Design review of the part shown in the three views and the two pictorial views. Dimensions are in mm from the part's minimum x, y and z. A direction names the side the tool comes from. Coordinates: 2 decimals unless noted, no trailing zeros. Loops run counter-clockwise (first coordinate to the right, second up) from the corner with the lowest first, then second, coordinate; pieces in that order, holes last. Notation, with made-up numbers: M 3,-6.75 L 22,-6.75 A12 ccw 22,16.25 Z; hole C 68.25,65.25 d4. An arc over 180 degrees is marked long. Answer as a JSON object with one key per item and string values. Group by question number.
Item 1: Mouldability with a two-part tool opening along X and no side actions: class the marked faces 3, 4, 5 and 6 as +X half, -X half, draft (parallel to the pull), parting line (faces both ways), or undercut.
Item 2: Add section A-A (x = 237). State the section outline as (y, z) points, then the cut area to 3 significant figures.
Item 3: Tool access review of the marked faces 1 and 2: name each direction out of +Z, -Z, +X, -X, +Y, -Y from which nothing blocks a thin tool from reaching the whole face with its end or side.
Item 4: Wall thickness on L1, parallel to X at y = 83, z = 149.5; L2, parallel to Y at x = 105, z = 110: over which ranges is each line inside the solid? List them lowest first. Write a range as from..to.
Item 5: Add section B-B (y = 100). State the section outline as (x, z) points, then the cut area to 3 significant figures.
Item 6: Add section C-C (z = 172). State the section outline as (x, y) points.
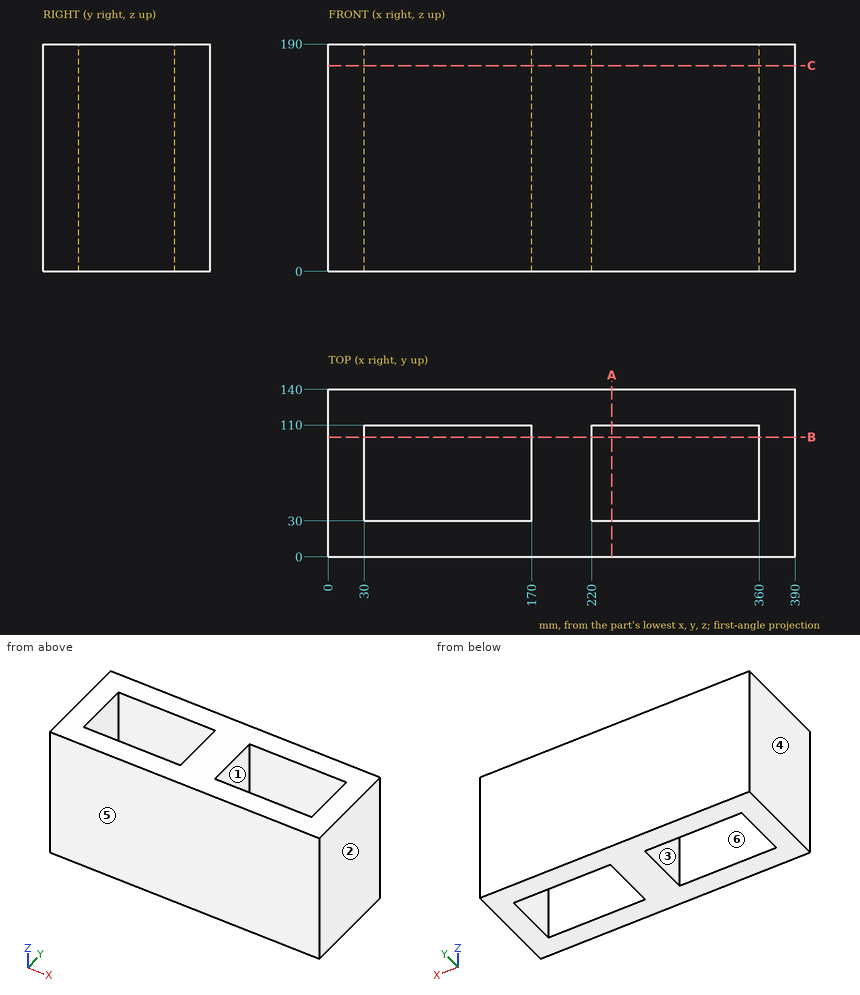
From the geometry:
{
 "1": {"face 3": "undercut", "face 4": "-X half", "face 5": "draft", "face 6": "undercut"},
 "2": {"outline": "M 0,0 L 30,0 L 30,190 L 0,190 Z; M 110,0 L 140,0 L 140,190 L 110,190 Z", "area": "11,400 mm²"},
 "3": {"face 1": "+Z, -Z", "face 2": "+Z, -Z, +X, +Y, -Y"},
 "4": {"L1": "x = 0..30, 170..220, 360..390", "L2": "y = 0..30, 110..140"},
 "5": {"outline": "M 0,0 L 30,0 L 30,190 L 0,190 Z; M 170,0 L 220,0 L 220,190 L 170,190 Z; M 360,0 L 390,0 L 390,190 L 360,190 Z", "area": "20,900 mm²"},
 "6": {"outline": "M 0,0 L 390,0 L 390,140 L 0,140 Z; hole M 30,30 L 170,30 L 170,110 L 30,110 Z; hole M 220,30 L 360,30 L 360,110 L 220,110 Z"}
}
